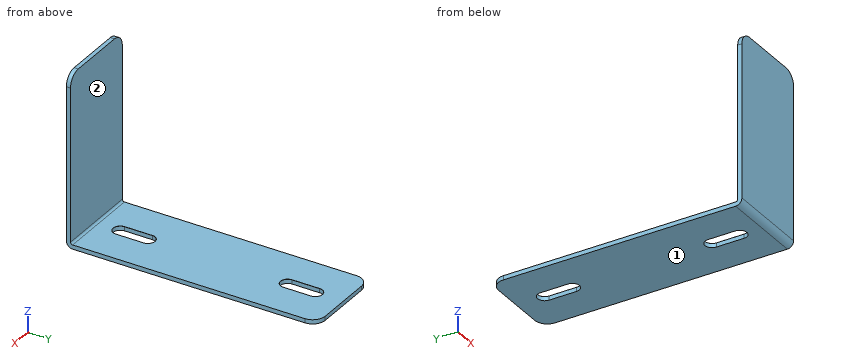
from build123d import *

# Parameters (mm, degrees)
SKETCH1_W                    = 20
SKETCH1_H                    = 60
BASE_FLANGE1_DEPTH           = 1
EDGE_FLANGE1_STRIP_W         = 5
EDGE_FLANGE1_STRIP_H         = 1
EDGE_FLANGE1_STRIP_CUT_DEPTH = 20
EDGE_FLANGE1_DEPTH           = 20
FILLET1_R                    = 3
M3_START                     = -1
M3_CLEARANCE_SLOT4_DEPTH     = 1


with BuildPart() as part:
    # Base-Flange1: sheet metal written as solids
    # Sketch1 → Base-Flange1 (new body)
    with BuildSketch(Plane.XY):
        Rectangle(SKETCH1_W, SKETCH1_H)
    extrude(amount=-BASE_FLANGE1_DEPTH)

    # Edge-Flange1: sheet metal written as solids
    # Edge-Flange1 strip (on a plane across the edge) → Edge-Flange1 strip cut (cut)
    with BuildSketch(Plane(origin=(-10, -30, 0), x_dir=(0, 1, 0), z_dir=(1, 0, 0))):
        with Locations((-1, -0.5)):
            Rectangle(EDGE_FLANGE1_STRIP_W, EDGE_FLANGE1_STRIP_H)
    extrude(amount=EDGE_FLANGE1_STRIP_CUT_DEPTH, mode=Mode.SUBTRACT)

    # Edge-Flange1 section (on a plane across the edge) → Edge-Flange1 (add)
    with BuildSketch(Plane(origin=(-10, -30, 0), x_dir=(0, 1, 0), z_dir=(1, 0, 0))):
        with BuildLine():
            Line((0, 0.5), (0, 40))
            Line((0, 40), (1, 40))
            Line((1, 40), (1, 0.5))
            ThreePointArc((1, 0.5), (1.146446609, 0.146446609), (1.5, 0))
            Line((1.5, 0), (1.5, -1))
            ThreePointArc((1.5, -1), (0.439339828, -0.560660172), (0, 0.5))
        make_face()
    extrude(amount=EDGE_FLANGE1_DEPTH)

    # Fillet1
    fillet1_edges = [part.edges().sort_by_distance(p)[0] for p in [
        (-10, -29.5, 40),
        (10, -29.5, 40),
        (-10, 30, -0.5),
        (10, 30, -0.5),
    ]]
    fillet(fillet1_edges, radius=FILLET1_R)

    # M3 Clearance Slot4: read off the stored shape, not the designer's step
    # M3 Clearance Slot4 outline → M3 Clearance Slot4 (cut)
    with BuildSketch(Plane.XY.offset(M3_START)):
        with BuildLine():
            Line((1.7, -23.3), (1.7, -16.7))
            ThreePointArc((1.7, -16.7), (0, -15), (-1.7, -16.7))
            Line((-1.7, -16.7), (-1.7, -23.3))
            ThreePointArc((-1.7, -23.3), (0, -25), (1.7, -23.3))
        make_face()
        with BuildLine():
            ThreePointArc((1.7, 23.3), (0, 25), (-1.7, 23.3))
            Line((-1.7, 23.3), (-1.7, 16.7))
            ThreePointArc((-1.7, 16.7), (0, 15), (1.7, 16.7))
            Line((1.7, 16.7), (1.7, 23.3))
        make_face()
    extrude(amount=M3_CLEARANCE_SLOT4_DEPTH, mode=Mode.SUBTRACT)

    # M3 Clearance Slot4 2: loft between two sections, ruled curve by curve
    m3_clearance_slot4_2_from = [
        Edge.make_three_point_arc((1.7, -16.7, -0.025), (1.202081528, -15.497918472, -0.025), (0, -15, -0.025)),
        Edge.make_three_point_arc((0, -15, -0.025), (-1.202081528, -15.497918472, -0.025), (-1.7, -16.7, -0.025)),
        Edge.make_three_point_arc((-1.7, -23.3, -0.025), (-1.202081528, -24.502081528, -0.025), (0, -25, -0.025)),
        Edge.make_three_point_arc((0, -25, -0.025), (1.202081528, -24.502081528, -0.025), (1.7, -23.3, -0.025)),
        Edge.make_line((-1.7, -16.7, -0.025), (-1.7, -23.3, -0.025)),
        Edge.make_line((1.7, -16.7, -0.025), (1.7, -23.3, -0.025)),
    ]
    m3_clearance_slot4_2_to = [
        Edge.make_three_point_arc((1.725, -16.7, 0), (1.219759198, -15.480240802, 0), (0, -14.975, 0)),
        Edge.make_three_point_arc((0, -14.975, 0), (-1.219759198, -15.480240802, 0), (-1.725, -16.7, 0)),
        Edge.make_three_point_arc((-1.725, -23.3, 0), (-1.219759198, -24.519759198, 0), (0, -25.025, 0)),
        Edge.make_three_point_arc((0, -25.025, 0), (1.219759198, -24.519759198, 0), (1.725, -23.3, 0)),
        Edge.make_line((-1.725, -16.7, 0), (-1.725, -23.3, 0)),
        Edge.make_line((1.725, -16.7, 0), (1.725, -23.3, 0)),
    ]
    m3_clearance_slot4_2 = Solid(Shell([*[Face.make_surface_from_curves(m3_clearance_slot4_2_from[k], m3_clearance_slot4_2_to[k]) for k in range(6)], Face(Wire(m3_clearance_slot4_2_from)), Face(Wire(m3_clearance_slot4_2_to))]))
    add(m3_clearance_slot4_2, mode=Mode.SUBTRACT)

    # M3 Clearance Slot4 3: loft between two sections, ruled curve by curve
    m3_clearance_slot4_3_from = [
        Edge.make_three_point_arc((1.7, 23.3, -0.025), (1.202081528, 24.502081528, -0.025), (0, 25, -0.025)),
        Edge.make_three_point_arc((0, 25, -0.025), (-1.202081528, 24.502081528, -0.025), (-1.7, 23.3, -0.025)),
        Edge.make_three_point_arc((-1.7, 16.7, -0.025), (-1.202081528, 15.497918472, -0.025), (0, 15, -0.025)),
        Edge.make_three_point_arc((0, 15, -0.025), (1.202081528, 15.497918472, -0.025), (1.7, 16.7, -0.025)),
        Edge.make_line((-1.7, 23.3, -0.025), (-1.7, 16.7, -0.025)),
        Edge.make_line((1.7, 23.3, -0.025), (1.7, 16.7, -0.025)),
    ]
    m3_clearance_slot4_3_to = [
        Edge.make_three_point_arc((1.725, 23.3, 0), (1.219759198, 24.519759198, 0), (0, 25.025, 0)),
        Edge.make_three_point_arc((0, 25.025, 0), (-1.219759198, 24.519759198, 0), (-1.725, 23.3, 0)),
        Edge.make_three_point_arc((-1.725, 16.7, 0), (-1.219759198, 15.480240802, 0), (0, 14.975, 0)),
        Edge.make_three_point_arc((0, 14.975, 0), (1.219759198, 15.480240802, 0), (1.725, 16.7, 0)),
        Edge.make_line((-1.725, 23.3, 0), (-1.725, 16.7, 0)),
        Edge.make_line((1.725, 23.3, 0), (1.725, 16.7, 0)),
    ]
    m3_clearance_slot4_3 = Solid(Shell([*[Face.make_surface_from_curves(m3_clearance_slot4_3_from[k], m3_clearance_slot4_3_to[k]) for k in range(6)], Face(Wire(m3_clearance_slot4_3_from)), Face(Wire(m3_clearance_slot4_3_to))]))
    add(m3_clearance_slot4_3, mode=Mode.SUBTRACT)


solid = part.part
Source: CAD feature listing. Evaluate the final solid. Frame: model axes, mm. Face numbers are marked on the shaded views. A direction names the side the tool comes from. Give positions to 0.01 mm unless a question says otherwise; leave off trailing zeros. Write each loop counter-clockwise with the first axis right and the second up, starting at its lowest first coordinate (ties: lowest second). Pieces come first, ordered by that corner, then holes. Notation, with made-up numbers: (33.25, 55.5) -> (89.25, 55.5) arc R12 cw to (89.25, 76.5) -> close; hole circle Ø11 at (44.25, 67.5). An arc over 180 degrees is marked (long way). Return JSON: item names as keys, results as strings. Group by question number.
1. Pin query (flat end, axial travel): pin 1 Ø2 at (x, y) = (4, 10) entering from +Z. Return the tip coordinate at first contact, or that it passes through.
2. Section A-A, the plane x = -3.5. Output: boundary loops of the cut face in (y, z), then the cut area to 3 significant figures.
3. Material intervals for line 1 (Y direction, x = -9, z = 2); line 2 (Z direction, x = -3.5, y = 8.5), sorted ascending. Write a range as from..to.
4. Section B-B, the plane z = 34. Output: boundary loops of the cut face in (x, y).
5. Section C-C, the plane y = 5.5. Output: boundary loops of the cut face in (x, z).
6. Access query for the marked faces 1 and 2. Directions: +Z, -Z, +X, -X, +Y, -Y. A direction counts if a zero-diameter tool reaches every point of the face in a straight line with its end or side. Return the directions, or none.
Determined:
{
 "1": {"pin 1": "stops at z = 0"},
 "2": {"outline": "(-30, 0.5) arc R1.5 ccw to (-28.5, -1) -> (30, -1) -> (30, 0) -> (-28.5, 0) arc R0.5 cw to (-29, 0.5) -> (-29, 40) -> (-30, 40) -> close", "area": "99.6 mm2"},
 "3": {"line 1": "y = -30..-29", "line 2": "z = -1..0"},
 "4": {"outline": "(-10, -30) -> (10, -30) -> (10, -29) -> (-10, -29) -> close"},
 "5": {"outline": "(-10, -1) -> (10, -1) -> (10, 0) -> (-10, 0) -> close"},
 "6": {"face 1": "-Z, +X, -X, +Y, -Y", "face 2": "+Z, +X, -X, +Y"}
}
